Check sheet for the drawn part. Datum: minimum x, y, z corner. Units: mm. A direction names the side the tool comes from. Round coordinates to 2 decimals unless told otherwise and drop trailing zeros. Order: outer loops, then holes, each group sorted by start corner. A loop starts at its lowest first (then second) coordinate and runs counter-clockwise, first axis right, second up. Notation, with made-up numbers: (48, -6.75) -> (53, -6.75) arc R19 cw to (53, 12.25) -> close; hole circle Ø11 at (56, 28.25). An arc over 180 degrees is marked (long way). Answer in a Markdown table with one row per item.
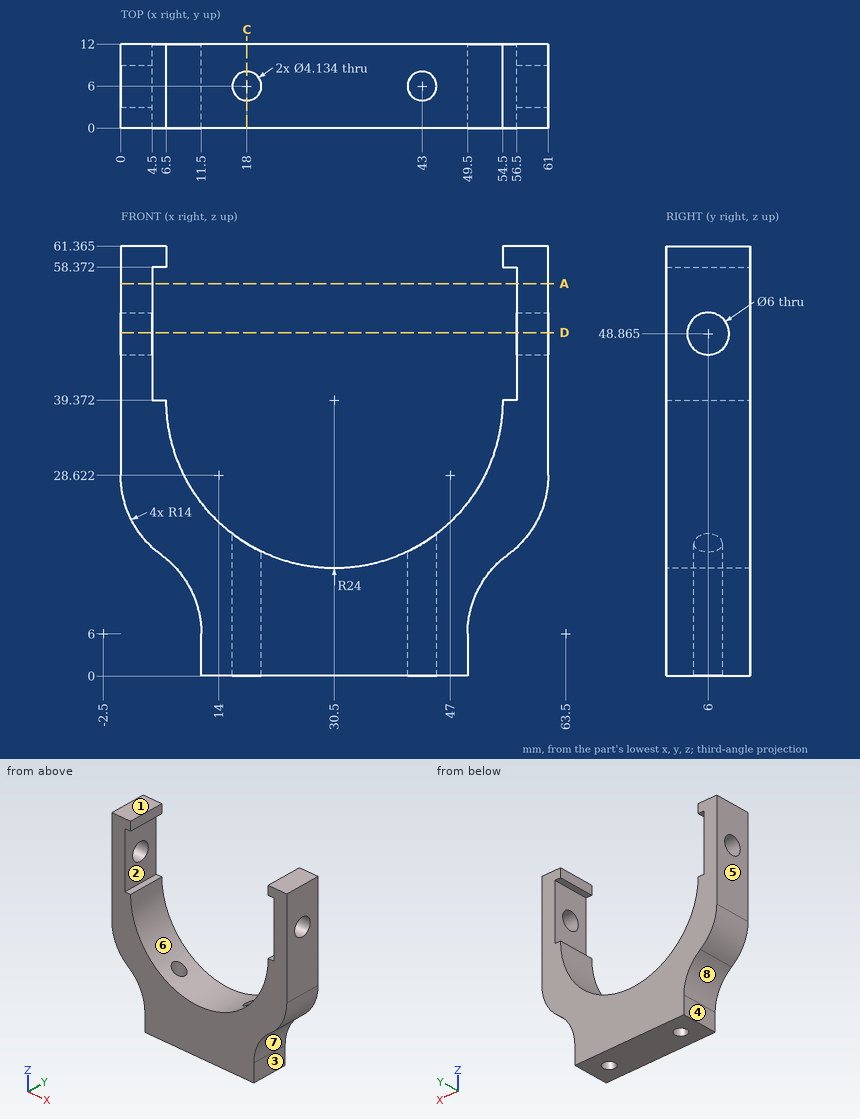
(1) Draft check along X on the marked faces 6, 7 and 8. Enter one of: pulls with the +X half, pulls with the -X half, needs draft (parallel to the pull), parting line crosses it, or undercut.
Solutions:
| item | result |
|---|---|
| face 6 | undercut |
| face 7 | pulls with the +X half |
| face 8 | pulls with the -X half |
(2) Depth check by flat-ended pin: pin 1 Ø5 at (x, y) = (26.5, 3) entering from +Z; pin 2 Ø2 at (x, y) = (56, 8.5) entering from -Z (1 decimal); pin 3 Ø5 at (y, z) = (9, 3.5) entering from -X. Enter the tip coordinate at first touch or a pass-through.
Solutions:
| item | result |
|---|---|
| pin 1 | z = 16.27 |
| pin 2 | z = 17.1 |
| pin 3 | x = 11.5 |
(3) Tool access check on the marked faces 1, 2, 3, 4 and 5. Record the directions out of +Z, -Z, +X, -X, +Y, -Y that give a thin tool (end or side, any length) a straight path to the whole face; none if there is none.
Solutions:
| item | result |
|---|---|
| face 1 | +Z, +X, -X, +Y, -Y |
| face 2 | +Y, -Y |
| face 3 | -Z, +X, +Y, -Y |
| face 4 | -Z, -X, +Y, -Y |
| face 5 | +Z, -Z, -X, +Y, -Y |
(4) Scan lines: probe 1 along X at (y, z) = (1, 54); probe 2 along X at (y, z) = (6, 13) (1 decimal); probe 3 along Y at (x, z) = (43, 12.25). Record each from-to range of solid material in increasing order. Write a range as from..to.
Solutions:
| item | result |
|---|---|
| probe 1 | 0..4.5, 56.5..61 |
| probe 2 | 9.6..15.9, 20.1..40.9, 45.1..51.4 |
| probe 3 | 0..3.93, 8.07..12 |
(5) Section check C-C on x = 18. Record the boundary of the cut face in (y, z), plus the area to 3 significant figures.
Solutions:
| item | result |
|---|---|
| outline | (0, 0) -> (3.93, 0) -> (3.93, 18.88) -> (0, 18.88) -> close; (8.07, 0) -> (12, 0) -> (12, 18.88) -> (8.07, 18.88) -> close |
| area | 149 mm^2 |
(6) Section check D-D on z = 49. Record the boundary of the cut face in (x, y).
Solutions:
| item | result |
|---|---|
| outline | (0, 0) -> (4.5, 0) -> (4.5, 3) -> (0, 3) -> close; (0, 9) -> (4.5, 9) -> (4.5, 12) -> (0, 12) -> close; (56.5, 0) -> (61, 0) -> (61, 3) -> (56.5, 3) -> close; (56.5, 9) -> (61, 9) -> (61, 12) -> (56.5, 12) -> close |
(7) Section check A-A on z = 56. Record the boundary of the cut face in (x, y), plus the area to 3 significant figures.
Solutions:
| item | result |
|---|---|
| outline | (0, 0) -> (4.5, 0) -> (4.5, 12) -> (0, 12) -> close; (56.5, 0) -> (61, 0) -> (61, 12) -> (56.5, 12) -> close |
| area | 108 mm^2 |
